```python
from build123d import *

# Parameters (mm, degrees)
SKETCH_1_W          = 22
SKETCH_1_H          = 16
SKETCH_1_W_2        = 19
SKETCH_1_H_2        = 13
EXTRUDE_1_DEPTH     = 23
SKETCH_2_W          = 22
SKETCH_2_H          = 16
EXTRUDE_2_DEPTH     = 3
SKETCH_3_R          = 1.25
CUT_EXTRUDE_1_DEPTH = 3
CHAMFER_1_SIZE      = 2
SKETCH_4_R          = 1.5
CUT_EXTRUDE_2_DEPTH = 28
CUT_EXTRUDE_3_DEPTH = 13


with BuildPart() as part:
    # Эскиз1 → Бобышка-Вытянуть1 (new body)
    with BuildSketch(Plane(origin=(0, 0, 0), x_dir=(1, 0, 0), z_dir=(0, 1, 0))):
        with Locations((-0.249343832, 2.073490814)):
            Rectangle(SKETCH_1_W, SKETCH_1_H)
        with Locations((-0.249343832, 2.073490814)):
            Rectangle(SKETCH_1_W_2, SKETCH_1_H_2, mode=Mode.SUBTRACT)
    extrude(amount=EXTRUDE_1_DEPTH)

    # Эскиз2 → Бобышка-Вытянуть2 (add)
    with BuildSketch(Plane.XZ):
        with Locations((-0.249343832, -2.073490814)):
            Rectangle(SKETCH_2_W, SKETCH_2_H)
    extrude(amount=EXTRUDE_2_DEPTH)

    # Эскиз3 → Вырез-Вытянуть1 (cut)
    with BuildSketch(Plane(origin=(0, 0, 0), x_dir=(1, 0, 0), z_dir=(0, 1, 0))):
        with Locations((-0.249343832, 2.073490814)):
            Circle(SKETCH_3_R)
    extrude(amount=-CUT_EXTRUDE_1_DEPTH, mode=Mode.SUBTRACT)

    # Фаска1
    chamfer_1_edges = [part.edges().sort_by_distance(p)[0] for p in [
        (-1.499343832, 0, -2.073490814),
    ]]
    chamfer(chamfer_1_edges, length=CHAMFER_1_SIZE)

    # Эскиз4 → Вырез-Вытянуть2 (cut)
    with BuildSketch(Plane(origin=(10.750656168, 0, 0), x_dir=(0, 0, -1), z_dir=(1, 0, 0))):
        with Locations((2.073490814, 1.5)):
            Circle(SKETCH_4_R)
    extrude(amount=-CUT_EXTRUDE_2_DEPTH, mode=Mode.SUBTRACT)

    # Эскиз5 → Вырез-Вытянуть3 (cut)
    with BuildSketch(Plane.XY.offset(-8.573490814)):
        Polygon((9.250656168, 23), (9.54509952, 19), (9.250656168, 15), align=None)
        Polygon((-10.043787184, 19), (-9.749343832, 15), (-9.749343832, 23), align=None)
    extrude(amount=CUT_EXTRUDE_3_DEPTH, mode=Mode.SUBTRACT)


solid = part.part
```
Could you check a few things on this model? Use its own coordinates, in mm. A direction names the side the tool comes from. Round coordinates to 2 decimals unless told otherwise and drop trailing zeros. Loops run counter-clockwise (first coordinate to the right, second up) from the corner with the lowest first, then second, coordinate; pieces in that order, holes last. Notation, with made-up numbers: (-3.75, 65) -> (35.25, 65) arc R20 cw to (35.25, 104) -> close; hole circle Ø5 at (-9.75, 60). An arc over 180 degrees is marked (long way). One line per question, with ' | ' between items.
(1) If we section it at A-A on y = 10.25: List the corners of the cut face in (x, z) for me, and give its area (3 significant figures).
Model answer:
outline: (-11.25, -10.07) -> (10.75, -10.07) -> (10.75, 5.93) -> (-11.25, 5.93) -> close; hole (-9.75, -8.57) -> (9.25, -8.57) -> (9.25, 4.43) -> (-9.75, 4.43) -> close | area: 105 mm^2
(2) For pin 1 Ø2.5 at (y, z) = (1.5, -2.07) entering from -X; pin 2 Ø6.5 at (x, z) = (1.5, -4.5) entering from +Y; pin 3 Ø3 at (x, z) = (-0.25, -2.07) entering from +Y, each with a flat end and sliding along its axis, tell me the tip position at first contact or that it passes through.
Model answer:
pin 1: passes through | pin 2: stops at y = 0 | pin 3: stops at y = -1.75
(3) If we section it at B-B on z = -7.25: List the corners of the cut face in (x, y) for me, and give its area (3 significant figures).
Model answer:
outline: (-11.25, -3) -> (10.75, -3) -> (10.75, 23) -> (9.25, 23) -> (9.55, 19) -> (9.25, 15) -> (9.25, 0) -> (-9.75, 0) -> (-9.75, 15) -> (-10.04, 19) -> (-9.75, 23) -> (-11.25, 23) -> close | area: 133 mm^2
(4) Thinking about a two-plate mould opening in Y: for faces 1 (the face through (-0.547, -1.875, -0.731)), 2 (the face through (-11.249, 10, -2)), 3 (the face through (-9.9, 17.03, -2.16)), which applies, released by +Y, released by -Y, zero draft, split by the parting line, or undercut?
Model answer:
face 1: released by +Y | face 2: zero draft | face 3: undercut
(5) If I drill on probe 1 along X at (y, z) = (6.5, -6.25); probe 2 along Z at (x, y) = (1.25, 17); probe 3 along Y at (x, z) = (7.5, 1), over which ranges is the centre line in solid material (lowest first)?
Model answer:
probe 1: x = -11.25 to -9.75, 9.25 to 10.75 | probe 2: z = -10.07 to -8.57, 4.43 to 5.93 | probe 3: y = -3 to 0
(6) If we section it at C-C on x = -9.25: List the corners of the cut face in (y, z) for me.
Model answer:
outline: (-3, -10.07) -> (23, -10.07) -> (23, -8.57) -> (0, -8.57) -> (0, 4.43) -> (23, 4.43) -> (23, 5.93) -> (-3, 5.93) -> close
(7) If we section it at D-D on y = 1.5: List the corners of the cut face in (x, z) for me, and give its area (3 significant figures).
Model answer:
outline: (-11.25, -10.07) -> (10.75, -10.07) -> (10.75, -3.57) -> (9.25, -3.57) -> (9.25, -8.57) -> (-9.75, -8.57) -> (-9.75, -3.57) -> (-11.25, -3.57) -> close; (-11.25, -0.57) -> (-9.75, -0.57) -> (-9.75, 4.43) -> (9.25, 4.43) -> (9.25, -0.57) -> (10.75, -0.57) -> (10.75, 5.93) -> (-11.25, 5.93) -> close | area: 96.0 mm^2
(8) For faces 4 (the face through (-9.895, 21.028, -2.164)), 5 (the face through (-9.749, 7, -2)), 6 (the face through (-0.52, -2.493, -0.853)), which set-ups out of +Z, -Z, +X, -X, +Y, -Y let a thin tool reach every point of the face, with its end or its side?
Model answer:
face 4: none | face 5: +Y | face 6: +Y, -Y
